from build123d import *

# Parameters (mm, degrees)
SKETCH1_R           = 3.625
SKETCH1_R_2         = 2.075
BOSS_EXTRUDE1_DEPTH = 2.41
SKETCH2_R           = 1
SKETCH2_R_2         = 0.5
BOSS_EXTRUDE3_DEPTH = 1.89
BOSS_EXTRUDE4_START = 4.3
SKETCH1_2_R         = 3.625
SKETCH1_2_R_2       = 2.075
BOSS_EXTRUDE4_DEPTH = 0.8
SKETCH3_R           = 3.625
SKETCH3_R_2         = 2.075
CUT_EXTRUDE1_DEPTH  = 1.3
SKETCH4_R           = 2.075
SKETCH4_R_2         = 1
BOSS_EXTRUDE5_DEPTH = 0.7
SKETCH5_R           = 2.075
SKETCH5_R_2         = 1
CUT_EXTRUDE2_DEPTH  = 1


with BuildPart() as part:
    # Sketch1 → Boss-Extrude1 (new body)
    with BuildSketch(Plane(origin=(0, 0, 0), x_dir=(1, 0, 0), z_dir=(0, 1, 0))):
        with Locations(Location((0, 0, 0), (0, 0, 270))):
            Circle(SKETCH1_R)
        with Locations(Location((0, 0, 0), (0, 0, 270))):
            Circle(SKETCH1_R_2, mode=Mode.SUBTRACT)
    extrude(amount=BOSS_EXTRUDE1_DEPTH)

    # Sketch2 → Boss-Extrude3 (add)
    with BuildSketch(Plane(origin=(0, 2.41, 0), x_dir=(1, 0, 0), z_dir=(0, 1, 0))):
        with BuildLine():
            Line((-10.6054557, -10.267177528), (-3.625, 0))
            ThreePointArc((-3.625, 0), (2.238819707, 2.851019347), (0.859585555, -3.521610097))
            Line((0.859585555, -3.521610097), (-7.459503317, -12.737599274))
            ThreePointArc((-7.459503317, -12.737599274), (-10.267690381, -13.075364593), (-10.6054557, -10.267177528))
        make_face()
        with Locations(Location((0, 0, 0), (0, 0, 270))):
            Circle(SKETCH2_R, mode=Mode.SUBTRACT)
        with Locations(Location((-9.032479508, -11.502388401, 0), (0, 0, 270))):
            Circle(SKETCH2_R_2, mode=Mode.SUBTRACT)
        with Locations(Location((-7.797268635, -9.92941221, 0), (0, 0, 270))):
            Circle(SKETCH2_R_2, mode=Mode.SUBTRACT)
        with Locations(Location((-6.562057762, -8.356436018, 0), (0, 0, 270))):
            Circle(SKETCH2_R_2, mode=Mode.SUBTRACT)
        with Locations(Location((-5.32684689, -6.783459826, 0), (0, 0, 270))):
            Circle(SKETCH2_R_2, mode=Mode.SUBTRACT)
        with Locations(Location((-4.091636017, -5.210483635, 0), (0, 0, 270))):
            Circle(SKETCH2_R_2, mode=Mode.SUBTRACT)
        with Locations(Location((-2.856425144, -3.637507443, 0), (0, 0, 270))):
            Circle(SKETCH2_R_2, mode=Mode.SUBTRACT)
    extrude(amount=BOSS_EXTRUDE3_DEPTH)

    # Sketch1<2> → Boss-Extrude4 (add)
    with BuildSketch(Plane(origin=(0, 0, 0), x_dir=(1, 0, 0), z_dir=(0, 1, 0)).offset(BOSS_EXTRUDE4_START)):
        with Locations(Location((0, 0, 0), (0, 0, 270))):
            Circle(SKETCH1_2_R)
        with Locations(Location((0, 0, 0), (0, 0, 270))):
            Circle(SKETCH1_2_R_2, mode=Mode.SUBTRACT)
    extrude(amount=BOSS_EXTRUDE4_DEPTH)

    # Sketch3 → Cut-Extrude1 (cut)
    with BuildSketch(Plane.XZ):
        with Locations(Location((0, 0, 0), (0, 0, 270))):
            Circle(SKETCH3_R)
        with Locations(Location((0, 0, 0), (0, 0, 270))):
            Circle(SKETCH3_R_2, mode=Mode.SUBTRACT)
    extrude(amount=-CUT_EXTRUDE1_DEPTH, mode=Mode.SUBTRACT)

    # Sketch4 → Boss-Extrude5 (add)
    with BuildSketch(Plane(origin=(0, 4.3, 0), x_dir=(1, 0, 0), z_dir=(0, 1, 0))):
        with Locations(Location((0, 0, 0), (0, 0, 90))):
            Circle(SKETCH4_R)
        with Locations(Location((0, 0, 0), (0, 0, 270))):
            Circle(SKETCH4_R_2, mode=Mode.SUBTRACT)
    extrude(amount=BOSS_EXTRUDE5_DEPTH)

    # Sketch5 → Cut-Extrude2 (cut)
    with BuildSketch(Plane.XZ.offset(-2.41)):
        with Locations(Location((0, 0, 0), (0, 0, 270))):
            Circle(SKETCH5_R)
        with Locations(Location((0, 0, 0), (0, 0, 270))):
            Circle(SKETCH5_R_2, mode=Mode.SUBTRACT)
    extrude(amount=-CUT_EXTRUDE2_DEPTH, mode=Mode.SUBTRACT)


solid = part.part
Geometry: final body of the model. Coordinates: model frame, mm. Coordinates: 2 decimals unless noted, no trailing zeros. Order: outer loops, then holes, each group sorted by start corner. A loop starts at its lowest first (then second) coordinate and runs counter-clockwise, first axis right, second up.
(1) Section query A-A (x = -0.5). Return the cut outline in (y, z).
(2) First-contact query: pin 1 (2 mm diameter, centred on x = -0.5, z = 0, fed in from -Y); pin 2 (2 mm diameter, centred on x = 0.5, z = 0, fed in from +Y); pin 3 (1 mm diameter, centred on y = 3.5, z = 4, fed in from -X). Flat tips, straight axial feed; report the tip coordinate or a pass-through.
(3) Section query C-C (y = 2.15). Return the cut outline in (x, z) (3 decimals).
(4) Section query B-B (z = -0.5). Return the cut outline in (x, y), plus the area to 3 significant figures.
(5) Material intervals for probe 1 along X at (y, z) = (2.75, 0) (3 decimals); probe 2 along X at (y, z) = (4, 0) (3 decimals); probe 3 along Z at (x, y) = (-0.5, 3.5), sorted ascending.
(6) Section query D-D (x = -8.75). Return the cut outline in (y, z).
(7) Draft query along Z for faces 1 (the face through (-10.233, 3.342, 13.102)), 2 (the face through (-6, 4.3, 7)), 3 (the face through (-7.05, 3.34, 8.25)). Return one class per face: pulls with the +Z half, pulls with the -Z half, needs draft (parallel to the pull), parting line crosses it, or undercut.
Solution:
1. outline: (1.3, -3.59) - (5.1, -3.59) - (5.1, -2.01) - (5, -2.01) - (5, -0.87) - (3.41, -0.87) - (3.41, -2.01) - (1.3, -2.01) - close; (1.3, 2.01) - (3.41, 2.01) - (3.41, 0.87) - (5, 0.87) - (5, 2.01) - (5.1, 2.01) - (5.1, 3.59) - (4.3, 3.59) - (4.3, 5.03) - (2.41, 5.03) - (2.41, 3.59) - (1.3, 3.59) - close
2. pin 1: stops at y = 3.41
2. pin 2: stops at y = 5
2. pin 3: stops at x = -6.68
3. outline: circle Ø7.25 at (0, 0); hole circle Ø4.15 at (0, 0)
4. outline: (-3.59, 1.3) - (-2.01, 1.3) - (-2.01, 3.41) - (-0.87, 3.41) - (-0.87, 5) - (-2.01, 5) - (-2.01, 5.1) - (-3.59, 5.1) - close; (0.87, 3.41) - (2.01, 3.41) - (2.01, 1.3) - (3.59, 1.3) - (3.59, 5.1) - (2.01, 5.1) - (2.01, 5) - (0.87, 5) - close
4. area: 15.6 mm2
5. probe 1: x = -3.625 to -2.075, 2.075 to 3.625
5. probe 2: x = -3.625 to -1, 1 to 3.625
5. probe 3: z = -3.59 to -0.87, 0.87 to 5.03
6. outline: (2.41, 7.54) - (4.3, 7.54) - (4.3, 11.09) - (2.41, 11.09) - close; (2.41, 11.91) - (4.3, 11.91) - (4.3, 13.48) - (2.41, 13.48) - close
7. face 1: parting line crosses it
7. face 2: needs draft
7. face 3: undercut
